Input: part model. Units: mm. Frame: model coordinates. Coordinates: 2 decimals unless noted, no trailing zeros. Order: outer loops, then holes, each group sorted by start corner. A loop starts at its lowest first (then second) coordinate and runs counter-clockwise, first axis right, second up. Notation, with made-up numbers: (-40, -38.5) -> (16, -38.5) arc R13 ccw to (16, -33.5) -> close; hole circle Ø6 at (-34.5, -26.5). An arc over 180 degrees is marked (long way). One line per item, written item: value. Start each with the question number.
from build123d import *

# Parameters (mm, degrees)
SKETCH2_R           = 25.4
BASE_CYLINDER_DEPTH = 19.05
SKETCH3_R           = 56.35625
AFT_FLANGE_DEPTH    = 9.525
BOLT_CIRCLE_D       = 2.8702
BOLT_CIRCLE_DEPTH   = 9.525
SKETCH20_W          = 71.924294246
SKETCH20_H          = 16.463903039
CUT_EXTRUDE2_DEPTH  = 152.4


with BuildPart() as part:
    # Sketch2 → Base Cylinder (new body)
    with BuildSketch(Plane(origin=(0, 0, 0), x_dir=(1, 0, 0), z_dir=(0, 1, 0))):
        Circle(SKETCH2_R)
    extrude(amount=BASE_CYLINDER_DEPTH)

    # Sketch3 → Aft Flange (add)
    with BuildSketch(Plane.XZ):
        Circle(SKETCH3_R)
    extrude(amount=-AFT_FLANGE_DEPTH)

    # Bolt Circle
    with Locations(Plane(origin=(0, 0, 0), x_dir=(-1, 0, 0), z_dir=(0, -1, 0))):
        with Locations((-25.81275, -44.708994483), (-44.708994483, -25.81275), (-51.6255, 0), (-44.708994483, 25.81275), (-25.81275, 44.708994483), (0, 51.6255), (25.81275, 44.708994483), (44.708994483, 25.81275), (51.6255, 0), (44.708994483, -25.81275), (25.81275, -44.708994483), (0, -51.6255)):
            Hole(BOLT_CIRCLE_D / 2, depth=BOLT_CIRCLE_DEPTH)

    # Sketch20 → Cut-Extrude2 (cut, symmetric)
    with BuildSketch(Plane.XY):
        with Locations((-3.698234988, 17.756951519)):
            Rectangle(SKETCH20_W, SKETCH20_H)
    extrude(amount=CUT_EXTRUDE2_DEPTH, both=True, mode=Mode.SUBTRACT)


solid = part.part
1) Pin query (flat end, axial travel): pin 1 Ø5 at (y, z) = (6, -16.5) entering from -X; pin 2 Ø3 at (y, z) = (3.5, -37) entering from -X; pin 3 Ø4 at (x, y) = (41, 4.5) entering from -Z. Return the tip coordinate at first contact, or that it passes through.
2) Section query A-A, the plane z = 0. Return the cut outline in (x, y) (3 decimals), plus the area to 3 significant figures.
3) Mould query, pull axis Z, two halves, no side actions, for faces 1 (the flat face through (-1, 9.525, 1)), 2 (the cylindrical face through (-56.3, 4.7, 2.5)), 3 (the cylindrical face through (46.035, 4.829, -25.263)). Classes: +Z half, -Z half, draft (parallel to the pull), parting line (faces both ways), or undercut.
4) Section query B-B, the plane x = 0. Return the cut outline in (y, z) (3 decimals).
5) Ray query, line 1 along Z through (x, y) = (0, 6); line 2 along X through (y, z) = (3.75, -26.5); line 3 along X through (y, z) = (1.75, 27). Return the intervals inside material, ascending. Write a range as from..to.
6) Section query D-D, the plane x = 21. Return the cut outline in (y, z) (3 decimals).
7) Section query C-C, the plane y = 7.25. State how many separate pieces and enclosed holes the cut face has, plus the area to 3 significant figures.
Entries:
1. pin 1: stops at x = -54.59
1. pin 2: stops at x = -43.77
1. pin 3: stops at z = -40.68
2. outline: (-56.356, 0) -> (-53.061, 0) -> (-53.061, 9.525) -> (-56.356, 9.525) -> close; (-50.19, 0) -> (50.19, 0) -> (50.19, 9.525) -> (-50.19, 9.525) -> close; (53.061, 0) -> (56.356, 0) -> (56.356, 9.525) -> (53.061, 9.525) -> close
2. area: 1,020 mm2
3. face 1: draft
3. face 2: parting line
3. face 3: undercut
4. outline: (0, -56.356) -> (9.525, -56.356) -> (9.525, -53.061) -> (0, -53.061) -> close; (0, -50.19) -> (9.525, -50.19) -> (9.525, 50.19) -> (0, 50.19) -> close; (0, 53.061) -> (9.525, 53.061) -> (9.525, 56.356) -> (0, 56.356) -> close
5. line 1: z = -56.36..-53.06, -50.19..50.19, 53.06..56.36
5. line 2: x = -49.74..-45.97, -43.45..43.45, 45.97..49.74
5. line 3: x = -49.47..-45.52, -43.9..43.9, 45.52..49.47
6. outline: (0, -52.297) -> (9.525, -52.297) -> (9.525, 52.297) -> (0, 52.297) -> close
7. separate pieces: 1
7. enclosed holes: 12
7. area: 9,900 mm2
